Answer from the drawing. Dimensions are ordinates in mm from the lowest x, y and z of the part. Round coordinates to 2 decimals unless told otherwise and drop trailing zeros. Write each loop counter-clockwise with the first axis right and the second up, starting at its lowest first coordinate (ties: lowest second). Pieces come first, ordered by that corner, then holes. Notation, with made-up numbers: (-25.5, 79.25) -> (30.5, 79.25) arc R23 ccw to (30.5, 90.25) -> close; hole circle Ø1 at (72, 0.5). An arc over 180 degrees is marked (long way). Return JSON: item names as keys, results as strings. Group by question number.
(1) A cutting plane is placed at B-B on x = 79.5. Give the vertices of the cut face in (y, z).
(2) A cutting plane is placed at A-A on z = 14.5. Give the vertices of the cut face in (x, y).
(3) Straight lines are drawn through the part: line 1 (Z direction, x = 82, y = 2.45); line 2 (Z direction, x = 64.5, y = 2.25); line 3 (X direction, y = 2.4, z = 5). For each, find the intervals that lie inside material, in ascending order.
(4) A cutting plane is placed at C-C on y = 2.1. Give the vertices of the cut face in (x, z), then the cut area to 3 significant figures.
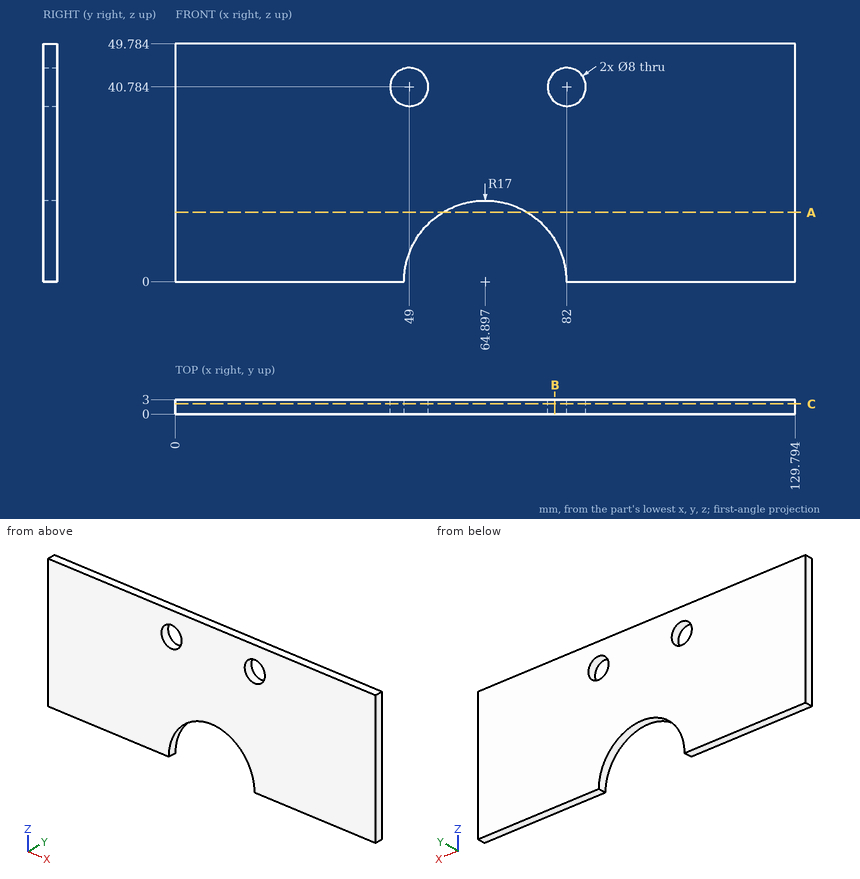
Checks:
{
 "1": {"outline": "(0, 8.7) -> (3, 8.7) -> (3, 37.66) -> (0, 37.66) -> close; (0, 43.91) -> (3, 43.91) -> (3, 49.78) -> (0, 49.78) -> close"},
 "2": {"outline": "(0, 0) -> (56.02, 0) -> (56.02, 3) -> (0, 3) -> close; (73.77, 0) -> (129.79, 0) -> (129.79, 3) -> (73.77, 3) -> close"},
 "3": {"line 1": "z = 0 to 36.78, 44.78 to 49.78", "line 2": "z = 17 to 49.78", "line 3": "x = 0 to 48.65, 81.15 to 129.79"},
 "4": {"outline": "(0, 0) -> (47.9, 0) arc R17 cw to (81.9, 0) -> (129.79, 0) -> (129.79, 49.78) -> (0, 49.78) -> close; hole circle Ø8 at (49, 40.78); hole circle Ø8 at (82, 40.78)", "area": "5,910 mm^2"}
}
